Work out the finished part from the listing and answer in its coordinate system (mm). Face numbers are marked on the shaded views. A direction names the side the tool comes from. Give positions to 0.01 mm unless a question says otherwise; leave off trailing zeros. Loops run counter-clockwise (first coordinate to the right, second up) from the corner with the lowest first, then second, coordinate; pieces in that order, holes last. Notation, with made-up numbers: (-27.5, -9) -> (21.5, -9) arc R15 ccw to (21.5, 4) -> close; hole circle Ø2 at (-35.5, -26). An arc over 180 degrees is marked (long way). Answer as CSV lines item,"result". Start each with the question number.
1. Determine the mould class of the marked faces 6, 7 and 8 for opening direction Z: +Z half, -Z half, draft (parallel to the pull), parting line (faces both ways), or undercut.
2. Find section C-C, the plane x = 33. Give the vertices of the cut face in (y, z), and give its area (3 significant figures).
3. Find section D-D, the plane z = -27. Give the vertices of the cut face in (x, y).
4. Find section A-A, the plane x = -11. Give the vertices of the cut face in (y, z), and give its area (3 significant figures).
5. Flat-ended cylindrical pins translate along their axes: pin 1 Ø1 at (x, y) = (-13.5, -10.5) entering from +Z; pin 2 Ø3.5 at (x, z) = (40.5, -17.5) entering from -Y; pin 3 Ø7.5 at (x, z) = (41.05, -18.5) entering from -Y; pin 4 Ø5 at (x, y) = (-38, -0.5) entering from +Z. Find the tip coordinate at first contact, or state that the pin passes through.
6. Find section B-B, the plane y = -15.5. Give the vertices of the cut face in (x, z), and give its area (3 significant figures).
7. Find the intervals of material crossed by line 1 along Z through (x, y) = (41, -21); line 2 along X through (y, z) = (8, 10); line 3 along X through (y, z) = (-5, -19.5), in increasing order.
8. A tool of negligible diameter and unlimited length cuts with its end or side. For the marked faces 1, 2, 3, 4 and 5, from which of +Z, -Z, +X, -X, +Y, -Y can it reach the whole face along a straight path? Write none if from no direction.
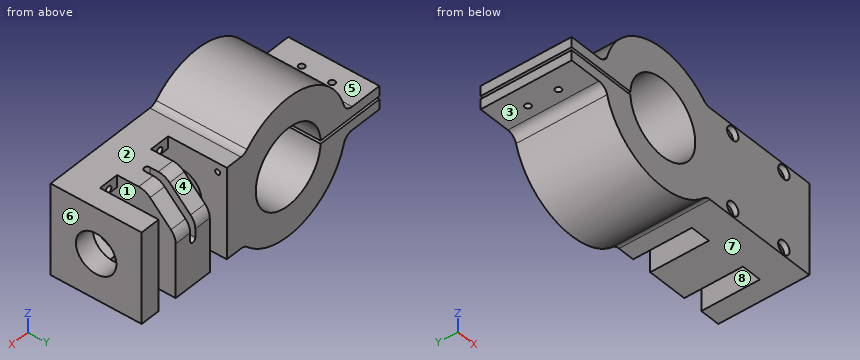
from build123d import *

# Parameters (mm, degrees)
BOSS_EXTRUDE1_DEPTH             = 22.5
F_3_0MM_DOWEL_HOLE1_D           = 3
BOSS_EXTRUDE2_START             = -8.493151603
BOSS_EXTRUDE2_OUTLINE_W         = 45
BOSS_EXTRUDE2_OUTLINE_H         = 45
BOSS_EXTRUDE2_DEPTH             = 60.493151603
SKETCH5_R                       = 10
CUT_EXTRUDE1_DEPTH              = 60
CUT_EXTRUDE2_START              = 22.5
SKETCH7_W                       = 10
SKETCH7_H                       = 45
CUT_EXTRUDE2_DEPTH              = 40
SKETCH8_W                       = 22.5
SKETCH8_H                       = 22.5
CUT_EXTRUDE3_DEPTH              = 1.5
CUT_EXTRUDE5_OUTLINE_W          = 1.5
CUT_EXTRUDE5_OUTLINE_H          = 12.613186919
CUT_EXTRUDE8_START              = 9.886859865
CUT_EXTRUDE8_DEPTH              = 12.613140135
CHAMFER1_SIZE                   = 15
FILLET3_R                       = 5
FILLET2_R                       = 8
BOSS_EXTRUDE3_DEPTH             = 40
M3X0_5_TAPPED_HOLE1_D           = 2.5
M3X0_5_TAPPED_HOLE1_DEPTH       = 25
M3X0_5_TAPPED_HOLE1_TIP         = 0.751075774
CBORE_FOR_M3_SBHCS1_D           = 3.4
CBORE_FOR_M3_SBHCS1_DEPTH       = 16
CBORE_FOR_M3_SBHCS1_CBORE_D     = 6.7
CBORE_FOR_M3_SBHCS1_CBORE_DEPTH = 2.65
CBORE_FOR_M3_SBHCS1_TIP         = 1.021463052


# Read off the part's stored shape, not the designer's step: Boss-Extrude2, Cut-Extrude5, Cut-Extrude8
with BuildPart() as part:
    # Sketch3 → Boss-Extrude1 (new, symmetric)
    with BuildSketch(Plane(origin=(0, 0, 0), x_dir=(1, 0, 0), z_dir=(0, 1, 0))):
        with BuildLine():
            Line((-53.560989258, 0.75), (-53.560989258, 5.75))
            Line((-53.560989258, 5.75), (-33.560989258, 5.75))
            ThreePointArc((-33.560989258, 5.75), (34.05, 0), (-33.560989258, -5.75))
            Line((-33.560989258, -5.75), (-53.560989258, -5.75))
            Line((-53.560989258, -5.75), (-53.560989258, -0.75))
            Line((-53.560989258, -0.75), (-19.035230495, -0.75))
            ThreePointArc((-19.035230495, -0.75), (19.05, 0), (-19.035230495, 0.75))
            Line((-19.035230495, 0.75), (-53.560989258, 0.75))
        make_face()
    extrude(amount=BOSS_EXTRUDE1_DEPTH, both=True)

    # Ø3.0mm Dowel Hole1 (through all)
    with Locations(Plane.XY.offset(5.75)):
        with Locations((-43.560989258, 7.5), (-43.560989258, -7.5)):
            Hole(F_3_0MM_DOWEL_HOLE1_D / 2)

    # Boss-Extrude2 outline → Boss-Extrude2 (add)
    with BuildSketch(Plane(origin=(34.05, 0, 0), x_dir=(0, 0, -1), z_dir=(1, 0, 0)).offset(BOSS_EXTRUDE2_START)):
        Rectangle(BOSS_EXTRUDE2_OUTLINE_W, BOSS_EXTRUDE2_OUTLINE_H)
    extrude(amount=BOSS_EXTRUDE2_DEPTH)

    # Sketch5 → Cut-Extrude1 (cut)
    with BuildSketch(Plane(origin=(86.05, 0, 0), x_dir=(0, 0, -1), z_dir=(1, 0, 0))):
        Circle(SKETCH5_R)
    extrude(amount=-CUT_EXTRUDE1_DEPTH, mode=Mode.SUBTRACT)

    # Sketch7 → Cut-Extrude2 (cut)
    with BuildSketch(Plane(origin=(0, 0, 0), x_dir=(1, 0, 0), z_dir=(0, 1, 0)).offset(CUT_EXTRUDE2_START)):
        with Locations((71.05, 0)):
            Rectangle(SKETCH7_W, SKETCH7_H)
        with Locations((41.05, 0)):
            Rectangle(SKETCH7_W, SKETCH7_H)
    extrude(amount=-CUT_EXTRUDE2_DEPTH, mode=Mode.SUBTRACT)

    # Sketch8 → Cut-Extrude3 (cut, symmetric)
    with BuildSketch(Plane(origin=(56.05, 0, 0), x_dir=(0, 0, -1), z_dir=(1, 0, 0))):
        with Locations((-11.25, 11.25)):
            Rectangle(SKETCH8_W, SKETCH8_H)
    extrude(amount=CUT_EXTRUDE3_DEPTH, both=True, mode=Mode.SUBTRACT)

    # Cut-Extrude5 outline → Cut-Extrude5 (revolve, cut)
    with BuildSketch(Plane(origin=(56.05, 0, 0), x_dir=(1, 0, 0), z_dir=(0, -1, 0))):
        with Locations((0.75, 16.19340654)):
            Rectangle(CUT_EXTRUDE5_OUTLINE_W, CUT_EXTRUDE5_OUTLINE_H)
    revolve(axis=Axis((56.05, 0, 0), (0, 0, 1)), mode=Mode.SUBTRACT)

    # Cut-Extrude8 outline → Cut-Extrude8 (cut)
    with BuildSketch(Plane(origin=(0, 0, 0), x_dir=(1, 0, 0), z_dir=(0, 1, 0)).offset(CUT_EXTRUDE8_START)):
        with BuildLine():
            ThreePointArc((57.55, 0), (56.05, 1.5), (54.55, 0))
            Line((54.55, 0), (57.55, 0))
        make_face()
    extrude(amount=CUT_EXTRUDE8_DEPTH, mode=Mode.SUBTRACT)

    # Chamfer1
    chamfer1_edges = [part.edges().sort_by_distance(p)[0] for p in [
        (61.8, 22.5, 22.5),
        (50.3, 22.5, 22.5),
    ]]
    chamfer(chamfer1_edges, length=CHAMFER1_SIZE)

    # Fillet3
    fillet3_edges = [part.edges().sort_by_distance(p)[0] for p in [
        (-33.560989258, 0, -5.75),
        (-33.560989258, 0, 5.75),
        (25.556848397, 0, -22.5),
        (25.556848397, 0, 22.5),
    ]]
    fillet(fillet3_edges, radius=FILLET3_R)

    # Fillet2
    fillet2_edges = [part.edges().sort_by_distance(p)[0] for p in [
        (50.3, 22.5, 7.5),
        (61.8, 22.5, 7.5),
        (50.3, 7.5, 22.5),
        (61.8, 7.5, 22.5),
    ]]
    fillet(fillet2_edges, radius=FILLET2_R)

    # Sketch15 → Boss-Extrude3 (add)
    with BuildSketch(Plane(origin=(36.05, 0, 0), x_dir=(0, 0, -1), z_dir=(1, 0, 0))):
        Polygon((-22.5, -6.5), (-16.5, -6.5), (-10.5, -17.5), (-22.5, -17.5), align=None)
        Polygon((22.5, -6.5), (16.5, -6.5), (10.5, -17.5), (22.5, -17.5), align=None)
    extrude(amount=BOSS_EXTRUDE3_DEPTH)

    # M3x0.5 Tapped Hole1
    with Locations(Plane(origin=(0, -22.5, 0), x_dir=(-1, 0, 0), z_dir=(0, -1, 0))):
        with Locations((-41.05, -18.5), (-71.05, 18.5), (-71.05, -18.5), (-41.05, 18.5)):
            Hole(M3X0_5_TAPPED_HOLE1_D / 2, depth=M3X0_5_TAPPED_HOLE1_DEPTH)
            with Locations((0, 0, -(M3X0_5_TAPPED_HOLE1_DEPTH + M3X0_5_TAPPED_HOLE1_TIP / 2))):  # 118° drill point
                Cone(0, M3X0_5_TAPPED_HOLE1_D / 2, M3X0_5_TAPPED_HOLE1_TIP, mode=Mode.SUBTRACT)

    # Sketch16 → M3x0.5 Tapped Hole2 (revolve, cut)
    with BuildSketch(Plane(origin=(46.05, 18, 18), x_dir=(0, 0, -1), z_dir=(0, 1, 0))):
        Polygon((0, 0), (0, 15.751075774), (1.25, 15), (1.25, 0), align=None)
    revolve(axis=Axis((52.4, 18, 18), (-1, 0, 0)), mode=Mode.SUBTRACT)

    # CBORE for M3 SBHCS1
    with Locations(Plane(origin=(0, -22.5, 0), x_dir=(-1, 0, 0), z_dir=(0, -1, 0))):
        with Locations((-71.05, 18.5), (-41.05, 18.5), (-41.05, -18.5), (-71.05, -18.5)):
            CounterBoreHole(CBORE_FOR_M3_SBHCS1_D / 2, CBORE_FOR_M3_SBHCS1_CBORE_D / 2, CBORE_FOR_M3_SBHCS1_CBORE_DEPTH, depth=CBORE_FOR_M3_SBHCS1_DEPTH)
            with Locations((0, 0, -(CBORE_FOR_M3_SBHCS1_DEPTH + CBORE_FOR_M3_SBHCS1_TIP / 2))):  # 118° drill point
                Cone(0, CBORE_FOR_M3_SBHCS1_D / 2, CBORE_FOR_M3_SBHCS1_TIP, mode=Mode.SUBTRACT)


solid = part.part
Resolved:
1,face 6,"draft"
1,face 7,"-Z half"
1,face 8,"undercut"
2,outline,"(-22.5, -22.5) -> (22.5, -22.5) -> (22.5, 22.5) -> (-22.5, 22.5) -> close; hole circle Ø20 at (0, 0); hole circle Ø2.5 at (18, 18)"
2,area,"1,710 mm^2"
3,outline,"(-20.75, -22.5) -> (20.75, -22.5) -> (20.75, 22.5) -> (-20.75, 22.5) -> close"
4,outline,"(-22.5, -32.22) -> (22.5, -32.22) -> (22.5, -15.55) -> (-22.5, -15.55) -> close; (-22.5, 15.55) -> (22.5, 15.55) -> (22.5, 32.22) -> (-22.5, 32.22) -> close"
4,area,"1,500 mm^2"
5,pin 1,"stops at z = 31.47"
5,pin 2,"stops at y = -19.85"
5,pin 3,"stops at y = -22.5"
5,pin 4,"stops at z = 6.19"
6,outline,"(-53.56, -5.75) -> (-37.54, -5.75) arc R5 cw to (-32.73, -9.37) arc R34.05 ccw to (24.17, -23.98) arc R5 cw to (27.72, -22.5) -> (86.05, -22.5) -> (86.05, 22.5) -> (27.72, 22.5) arc R5 cw to (24.17, 23.98) arc R34.05 ccw to (-32.73, 9.37) arc R5 cw to (-37.54, 5.75) -> (-53.56, 5.75) -> (-53.56, 0.75) -> (-19.04, 0.75) arc R19.05 cw (long way) to (-19.04, -0.75) -> (-53.56, -0.75) -> close; hole (36.05, -11.59) -> (46.05, -11.59) -> (46.05, 11.59) -> (36.05, 11.59) -> close; hole circle Ø3.4 at (41.05, -18.5); hole circle Ø3.4 at (41.05, 18.5); hole (66.05, -11.59) -> (76.05, -11.59) -> (76.05, 11.59) -> (66.05, 11.59) -> close; hole circle Ø3.4 at (71.05, -18.5); hole circle Ø3.4 at (71.05, 18.5)"
6,area,"4,640 mm^2"
7,line 1,"z = -22.5 to -21.85, -15.15 to 15.15, 21.85 to 22.5"
7,line 2,"x = -32.55 to -16.21, 16.21 to 36.05, 46.05 to 54.55, 57.55 to 66.05, 76.05 to 86.05"
7,line 3,"x = -27.91 to 36.05, 46.05 to 66.05, 76.05 to 86.05"
8,face 1,"+Y"
8,face 2,"+Z, +X, +Y, -Y"
8,face 3,"-Z, -X, +Y, -Y"
8,face 4,"+Z, +Y"
8,face 5,"+Z, -X, +Y, -Y"
